Autodesk Inventor part; units mm, degrees
ref_plane "Work Plane2" through (0, 0, 224.6312) normal (0, 0, 1) x (1, 0, 0)
ref_plane "YZ Plane" through (0, 0, 0) normal (1, 0, 0) x (0, 1, 0)
ref_plane "XZ Plane" through (0, 0, 0) normal (0, 1, 0) x (-1, 0, 0)
sketch "Sketch1" plane through (0, 0, 0) normal (0, 0, 1) x (1, 0, 0)
  circle A0 centre (0, 0) radius 431.8
  circle A1 centre (0, 0) radius 412.75
  dimension "d0" = 863.6
  dimension "d1" = 825.5
extrude "Extrusion1" add sketch "Sketch1" along normal blind 256.3812
chamfer "Chamfer1" distance 17.4625 angle 37.5 1 edges at (-431.8, 0, 0) measured on face at (-425.2038, 4.7488, 0)
ref_plane "Work Plane2" through (0, 0, 224.6312) normal (0, 0, 1) x (1, 0, 0)
ref_plane "Work Plane1" through (0, 0, 205.5812) normal (0, 0, 1) x (1, 0, 0)
split_face "Split1"
split_face "Split2"
chamfer "Chamfer2" distance 0.7937 angle 45 1 edges at (-412.75, 0, 256.3812)
properties part number "A1-19037-200-03 34in pipe" material "Steel, Mild"
Verification items for the finished model (mm, model axes). Give positions to 0.01 mm unless a question says otherwise; leave off trailing zeros. Loops run counter-clockwise (first coordinate to the right, second up) from the corner with the lowest first, then second, coordinate; pieces in that order, holes last.
1. Release check for a two-part mould opening along X. For faces 1 (the conical face through (-90.06, -405.55, 0.84)), 2 (the cylindrical face through (-327.544, 251.152, 126.005)), 3 (the flat face through (350, -222, 256.381)) record: +X half, -X half, draft (parallel to the pull), parting line (faces both ways), or undercut.
Derived:
face 1: parting line
face 2: undercut
face 3: draft
2. Cross-section at C-C on z = 218. Record the cut outline in (x, y), and give its area (3 significant figures).
Derived:
outline: circle Ø863.6 at (0, 0); hole circle Ø825.5 at (0, 0)
area: 50,500 mm2
3. Go/stop test with flat-tipped pins: P1, Ø1.5, axis at y = 239, z = 205.5, coming from the +X side; P2, Ø12, axis at y = 255, z = 188, coming from the +X side; P3, Ø12, axis at y = 205, z = 105.5, coming from the +X side. Record where each tip stops, or that it passes through.
Derived:
P1: stops at x = 360.12
P2: stops at x = 352.78
P3: stops at x = 383.21
4. Cross-section at A-A on y = 0. Record the cut outline in (x, z).
Derived:
outline: (-431.8, 13.4) - (-414.34, 0) - (-412.75, 0) - (-412.75, 255.59) - (-413.54, 256.38) - (-431.8, 256.38) - close; (412.75, 0) - (414.34, 0) - (431.8, 13.4) - (431.8, 256.38) - (413.54, 256.38) - (412.75, 255.59) - close
5. Material ranges on probe 1 along Y at (x, z) = (0, 113.5); probe 2 along Y at (x, z) = (365, 12); probe 3 along X at (y, z) = (-278, 55.5), recorded low to high.
Derived:
probe 1: y = -431.8 to -412.75, 412.75 to 431.8
probe 2: y = -227.28 to -192.71, 192.71 to 227.28
probe 3: x = -330.4 to -305.09, 305.09 to 330.4
